Check sheet for the modelled part. Datum: model origin and axes. Units: mm. A direction names the side the tool comes from. Coordinates: 2 decimals unless noted, no trailing zeros. Loops run counter-clockwise (first coordinate to the right, second up) from the corner with the lowest first, then second, coordinate; pieces in that order, holes last. Notation, with made-up numbers: M 7.5,71 L 66.5,71 A9 ccw 66.5,88 Z; hole C 47.25,78 d8. An arc over 180 degrees is marked long. Answer as CSV lines item,"result". Start each with the question number.
from build123d import *
from build123d.topology import SkipClean

# Parameters (mm, degrees)
BOSS_EXTRUDE1_DEPTH = 10
SKETCH3_W           = 5
SKETCH3_H           = 4
CUT_EXTRUDE1_DEPTH  = 74
BOSS_EXTRUDE2_DEPTH = 8
BOSS_EXTRUDE3_START = 5
SKETCH5_R           = 15
BOSS_EXTRUDE3_DEPTH = 5
SKETCH6_R           = 6
CUT_EXTRUDE2_DEPTH  = 13
RIB1_START          = -5
RIB1_DEPTH          = 10
SKETCH8_R           = 6
CUT_EXTRUDE4_DEPTH  = 11


# Read off the part's stored shape, not the designer's step: Rib1
with BuildPart() as part:
    # Sketch1 → Boss-Extrude1 (new body)
    with BuildSketch(Plane(origin=(0, 0, 0), x_dir=(1, 0, 0), z_dir=(0, 1, 0))):
        with BuildLine():
            Line((-36, 17.5), (36, 17.5))
            Line((36, 17.5), (36, -5.5))
            ThreePointArc((36, -5.5), (32.485281374, -13.985281374), (24, -17.5))
            Line((24, -17.5), (-24, -17.5))
            ThreePointArc((-24, -17.5), (-32.485281374, -13.985281374), (-36, -5.5))
            Line((-36, -5.5), (-36, 17.5))
        make_face()
    extrude(amount=BOSS_EXTRUDE1_DEPTH)

    # Sketch3 → Cut-Extrude1 (cut)
    with BuildSketch(Plane.ZY.offset(36)):
        with Locations((-15, 8)):
            Rectangle(SKETCH3_W, SKETCH3_H)
    extrude(amount=-CUT_EXTRUDE1_DEPTH, mode=Mode.SUBTRACT)

    # Sketch4 → Boss-Extrude2 (add)
    with BuildSketch(Plane(origin=(0, 0, -12.5), x_dir=(-1, 0, 0), z_dir=(0, 0, -1))):
        with BuildLine():
            Line((15, 60), (15, 23.747727085))
            ThreePointArc((15, 23.747727085), (17.450099602, 15.531888722), (24, 10))
            Line((24, 10), (-24, 10))
            ThreePointArc((-24, 10), (-17.450099602, 15.531888722), (-15, 23.747727085))
            Line((-15, 23.747727085), (-15, 60))
            ThreePointArc((-15, 60), (0, 75), (15, 60))
        make_face()
    extrude(amount=-BOSS_EXTRUDE2_DEPTH)

    # Sketch5 → Boss-Extrude3 (add)
    with SkipClean():  # the faces are left unmerged after this step: merging them gives an invalid solid
        with BuildSketch(Plane(origin=(0, 0, -12.5), x_dir=(-1, 0, 0), z_dir=(0, 0, -1)).offset(BOSS_EXTRUDE3_START)):
            with Locations((0, 60)):
                Circle(SKETCH5_R)
        extrude(amount=-BOSS_EXTRUDE3_DEPTH)

    # Sketch6 → Cut-Extrude2 (cut)
    with SkipClean():  # the faces are left unmerged after this step: merging them gives an invalid solid
        with BuildSketch(Plane(origin=(0, 0, -17.5), x_dir=(-1, 0, 0), z_dir=(0, 0, -1))):
            with Locations((0, 60)):
                Circle(SKETCH6_R)
        extrude(amount=-CUT_EXTRUDE2_DEPTH, mode=Mode.SUBTRACT)

    # Rib1 outline → Rib1 (add)
    with SkipClean():  # the faces are left unmerged after this step: merging them gives an invalid solid
        with BuildSketch(Plane(origin=(0, 0, 0), x_dir=(0, 0, -1), z_dir=(1, 0, 0)).offset(RIB1_START)):
            Polygon((4.5, 50), (-17.5, 10), (4.5, 10), align=None)
        extrude(amount=RIB1_DEPTH)

    # Sketch8 → Cut-Extrude4 (cut)
    with SkipClean():  # the faces are left unmerged after this step: merging them gives an invalid solid
        with BuildSketch(Plane(origin=(0, 10, 0), x_dir=(1, 0, 0), z_dir=(0, 1, 0))):
            with Locations(Location((24, -5.5, 0), (0, 0, 270))):
                Circle(SKETCH8_R)
            with Locations(Location((-24, -5.5, 0), (0, 0, 90))):
                Circle(SKETCH8_R)
        extrude(amount=-CUT_EXTRUDE4_DEPTH, mode=Mode.SUBTRACT)


solid = part.part
Item 1: Go/stop test with flat-tipped pins: pin 1 (6.5 mm diameter, centred on y = 39, z = -10.5, fed in from +X); pin 2 (12 mm diameter, centred on x = 20, z = 7.5, fed in from +Y); pin 3 (2 mm diameter, centred on y = 40.5, z = -11, fed in from -X); pin 4 (6.5 mm diameter, centred on y = 36, z = 8, fed in from -X). Record where each tip stops, or that it passes through.
Item 2: Set-up check for faces 4 (the face through (-5, 21, 2)), 5 (the face through (5, 21, 2)), 6 (the face through (-15, 42, -9)): record each of +Z, -Z, +X, -X, +Y, -Y from which the full face is reachable in a straight line by a thin tool's end or side.
Item 3: Sectioned sample at A-A, the plane x = 0. Record the boundary of the cut face in (y, z), and give its area (3 significant figures).
Item 4: Sectioned sample at B-B, the plane z = -8.5. Record the boundary of the cut face in (x, y), and give its area (3 significant figures).
Item 5: Sectioned sample at D-D, the plane z = 9. Record the boundary of the cut face in (x, y).
Item 6: Material ranges on line 1 (X direction, y = 6, z = 5); line 2 (Y direction, x = 0, z = -14); line 3 (Y direction, x = -12.5, z = 10.5), recorded low to high. Write a range as from..to.
Item 7: Sectioned sample at C-C, the plane y = 53. Record the boundary of the cut face in (x, z), and give its area (3 significant figures).
Item 8: Release check for a two-part mould opening along Y. For faces 1 (the face through (-36, 5, -6)), 2 (the face through (17, 10, 2)), 3 (the face through (4.42, 64.06, -11.09)) record: released by +Y, released by -Y, zero draft, split by the parting line, or undercut.
Reply:
1,pin 1,"x = 15"
1,pin 2,"y = 10"
1,pin 3,"x = -15"
1,pin 4,"through"
2,face 4,"+Z, -X, +Y"
2,face 5,"+Z, +X, +Y"
2,face 6,"+Z, -Z, -X, +Y"
3,outline,"M 0,-17.5 L 6,-17.5 L 6,-12.5 L 45,-12.5 L 45,-17.5 L 54,-17.5 L 54,-4.5 L 50,-4.5 L 10,17.5 L 0,17.5 Z; M 66,-17.5 L 75,-17.5 L 75,-4.5 L 66,-4.5 Z"
3,area,"1,280 mm²"
4,outline,"M -36,0 L 36,0 L 36,10 L 24,10 A15 cw 15,23.75 L 15,60 A15 ccw -15,60 L -15,23.75 A15 cw -24,10 L -36,10 Z; hole C 0,60 d12"
4,area,"2,530 mm²"
5,outline,"M -35.48,0 L -28.87,0 L -28.87,10 L -35.48,10 Z; M -19.13,0 L 19.13,0 L 19.13,10 L 5,10 L 5,25.45 L -5,25.45 L -5,10 L -19.13,10 Z; M 28.87,0 L 35.48,0 L 35.48,10 L 28.87,10 Z"
6,line 1,"-36..-29.98, -18.02..18.02, 29.98..36"
6,line 2,"0..6, 45..54, 66..75"
6,line 3,"0..10"
7,outline,"M -15,-12.5 L -13.27,-12.5 L -13.27,-17.5 L 13.27,-17.5 L 13.27,-12.5 L 15,-12.5 L 15,-4.5 L -15,-4.5 Z"
7,area,"373 mm²"
8,face 1,"zero draft"
8,face 2,"released by +Y"
8,face 3,"undercut"
